Source: CAD feature listing. Evaluate the final solid. Frame: model axes, mm. Face numbers are marked on the shaded views. Give positions to 0.01 mm unless a question says otherwise; leave off trailing zeros. Loops run counter-clockwise (first coordinate to the right, second up) from the corner with the lowest first, then second, coordinate; pieces in that order, holes last.
Autodesk Inventor part; units mm, degrees
ref_plane "YZ Plane" through (0, 0, 0) normal (1, 0, 0) x (0, 1, 0)
ref_plane "XZ Plane" through (0, 0, 0) normal (0, 1, 0) x (-1, 0, 0)
ref_plane "XY Plane" through (0, 0, 0) normal (0, 0, 1) x (1, 0, 0)
sketch "Sketch1" plane through (0, 0, 0) normal (0, 1, 0) x (-1, 0, 0)
  line L0 (0, 0) -> (-30, 0)
  line L1 (0, 0) -> (30, 0)
  line L2 (30, 0) -> (30, -100)
  line L3 (30, -100) -> (-30, -100)
  line L4 (-30, -100) -> (-30, 0)
  circle A0 centre (17, -85) radius 5.5
  circle A1 centre (17, -50) radius 5.5
  circle A2 centre (17, -15) radius 5.5
  circle A3 centre (-17, -15) radius 5.5
  circle A4 centre (-17, -50) radius 5.5
  circle A5 centre (-17, -85) radius 5.5
  arc A6 (-3, -87.7691) -> (3, -87.7691) centre (0, -87.7691) ccw
  arc A7 (3, -43.7691) -> (-3, -43.7691) centre (0, -43.7691) ccw
  line L5 (3, -87.7691) -> (3, -43.7691)
  line L6 (-3, -87.7691) -> (-3, -43.7691)
  dimension "d0" = 30
  dimension "d1" = 30
  dimension "d2" = 100
  dimension "d3" = 11
  dimension "d4" = 11
  dimension "d5" = 11
  dimension "d6" = 11
  dimension "d7" = 11
  dimension "d8" = 11
  dimension "d9" = 15
  dimension "d10" = 35
  dimension "d11" = 70
  dimension "d12" = 13
  dimension "d13" = 6
  dimension "d14" = 6
  dimension "d15" = 44
  dimension "d16" = 13
extrude "Extrusion1" add sketch "Sketch1" along normal blind 6
sketch "Sketch2" plane through (0, 6, 0) normal (0, 1, 0) x (1, 0, 0)
  line L0 (-30, 100) -> (-30, 0)
  line L1 (30, 0) -> (30, 100)
  line L2 (-30, 100) -> (30, 100)
  line L3 (30, 100) -> (30, 0)
  line L4 (-30, 0) -> (30, 0)
  line L5 (-30, 0) -> (-30, 100)
  circle A0 centre (-17, 85) radius 3.2
  circle A1 centre (-17, 15) radius 3.2
  circle A2 centre (17, 15) radius 3.2
  circle A3 centre (17, 50) radius 3.2
  circle A4 centre (17, 85) radius 3.2
  circle A5 centre (-17, 50) radius 3.2
  line L6 (-3, 43.7691) -> (-3, 87.7691)
  line L7 (-3, 87.7691) -> (-3, 43.7691)
  line L8 (3, 87.7691) -> (3, 43.7691)
  line L9 (3, 87.7691) -> (3, 43.7691)
  arc A6 (3, 87.7691) -> (-3, 87.7691) centre (0, 87.7691) ccw
  arc A7 (-3, 43.7691) -> (3, 43.7691) centre (0, 43.7691) ccw
  arc A8 (-3, 43.7691) -> (3, 43.7691) centre (0, 43.7691) ccw
  point P0 (0, 0)
  dimension "d19" = 6.4
  dimension "d21" = 6.4
  dimension "d22" = 6.4
  dimension "d23" = 6.4
  dimension "d24" = 6.4
  dimension "d25" = 15
  dimension "d26" = 35
  dimension "d27" = 70
  dimension "d28" = 13
  dimension "d29" = 13
  dimension "d30" = 6.4
  dimension "d31" = 6
extrude "Extrusion2" add sketch "Sketch2" along normal blind 14
sketch "Sketch4" plane through (30, 20, -100) normal (0, 0, -1) x (-1, 0, 0)
  circle A0 centre (20, -10) radius 4
  circle A1 centre (40, -10) radius 4
  line L0 (0, 0) -> (60, 0)
  line L1 (0, -20) -> (0, 0)
  line L2 (60, -20) -> (60, 0)
  point P0 (30, -20)
  point P1 (0, -25)
  point P2 (60, -25)
  dimension "d43" = 8
  dimension "d44" = 8
  dimension "d45" = 10
  dimension "d46" = 20
  dimension "d47" = 20
hole "Hole1" at (-10, 10, -100) at (10, 10, -100) direction (0, 0, 1) diameter 8 depth 12 tip angle 118
sketch "Sketch5" plane through (0, 20, 0) normal (0, 1, 0) x (1, 0, 0)
  line L0 (30, 100) -> (-30, 100)
  line L1 (30, 0) -> (30, 100)
  line L2 (30, 100) -> (30, 0)
  line L3 (30, 0) -> (25, 0)
  line L4 (-30, 0) -> (30, 0)
  line L5 (25, 0) -> (25, 100)
  line L6 (25, 100) -> (30, 100)
  line L7 (-30, 100) -> (-30, 0)
  line L8 (-30, 100) -> (-30, 0)
  line L9 (-30, 0) -> (-25, 0)
  line L10 (-25, 0) -> (-25, 100)
  line L11 (-30, 100) -> (-25, 100)
  point P0 (0, 0)
  dimension "d55" = 100
  dimension "d56" = 5
  dimension "d57" = 100
  dimension "d58" = 5
extrude "Extrusion4" add sketch "Sketch5" along normal blind 5 contours L1 L3 L5 L0 | L10 L4 L7 L0
chamfer "Chamfer1" distance 2 angle 45 1 edges at (-30, 0, -50) measured on face at (27.5, 0, -50)
chamfer "Chamfer2" distance 2 angle 45 1 edges at (30, 0, -50) measured on face at (27.5, 0, -50)
properties part number "Schneidführungs"
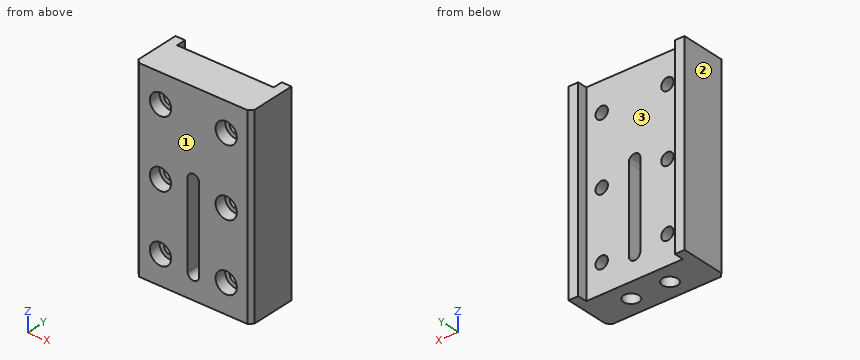
1) Cut plane A-A (x = 17). Return loops of the section in (y, z), and give its area (3 significant figures).
Checks:
outline: (0, -100) - (20, -100) - (20, -88.2) - (6, -88.2) - (6, -90.5) - (0, -90.5) - close; (0, -79.5) - (6, -79.5) - (6, -81.8) - (20, -81.8) - (20, -53.2) - (6, -53.2) - (6, -55.5) - (0, -55.5) - close; (0, -44.5) - (6, -44.5) - (6, -46.8) - (20, -46.8) - (20, -18.2) - (6, -18.2) - (6, -20.5) - (0, -20.5) - close; (0, -9.5) - (6, -9.5) - (6, -11.8) - (20, -11.8) - (20, 0) - (0, 0) - close
area: 1,530 mm2
2) Ray query, probe 1 along X at (y, z) = (10, -94.5); probe 2 along Z at (x, y) = (17, 13.5); probe 3 along X at (y, z) = (16.5, -15). Return the intervals inside material, ascending.
Checks:
probe 1: x = -30 to -14, -6 to 6, 14 to 30
probe 2: z = -100 to -88.2, -81.8 to -53.2, -46.8 to -18.2, -11.8 to 0
probe 3: x = -30 to -20.2, -13.8 to 13.8, 20.2 to 30
3) Cut plane C-C (y = 21). Return loops of the section in (x, z).
Checks:
outline: (-30, -100) - (-25, -100) - (-25, 0) - (-30, 0) - close; (25, -100) - (30, -100) - (30, 0) - (25, 0) - close
4) Cut plane D-D (x = 0). Return loops of the section in (y, z).
Checks:
outline: (0, -100) - (20, -100) - (20, -90.77) - (0, -90.77) - close; (0, -40.77) - (20, -40.77) - (20, 0) - (0, 0) - close
5) Contact query for flat-ended pins moving along their axis: P1, Ø3.5, axis at x = 18, z = -47.5, coming from the -Y side; P2, Ø25, axis at x = -7, z = -68.5, coming from the +Y side; P3, Ø3, axis at x = -12.5, y = 9.5, coming from the -Z side; P4, Ø5, axis at x = 17, z = -15, coming from the -Y side. Output: stop coordinate, or through.
Checks:
P1: stops at y = 6
P2: stops at y = 20
P3: stops at z = -100
P4: passes through
6) Cut plane B-B (z = -76). Return loops of the section in (x, y), and give its area (3 significant figures).
Checks:
outline: (-30, 2) - (-28, 0) - (-3, 0) - (-3, 20) - (-25, 20) - (-25, 25) - (-30, 25) - close; (3, 0) - (28, 0) - (30, 2) - (30, 25) - (25, 25) - (25, 20) - (3, 20) - close
area: 1,130 mm2
7) Pull-direction query (X, two-part tool) for the marked faces 1, 2 and 3; classes: released by +X, released by -X, zero draft, split by the parting line, or undercut.
Checks:
face 1: zero draft
face 2: released by -X
face 3: undercut
